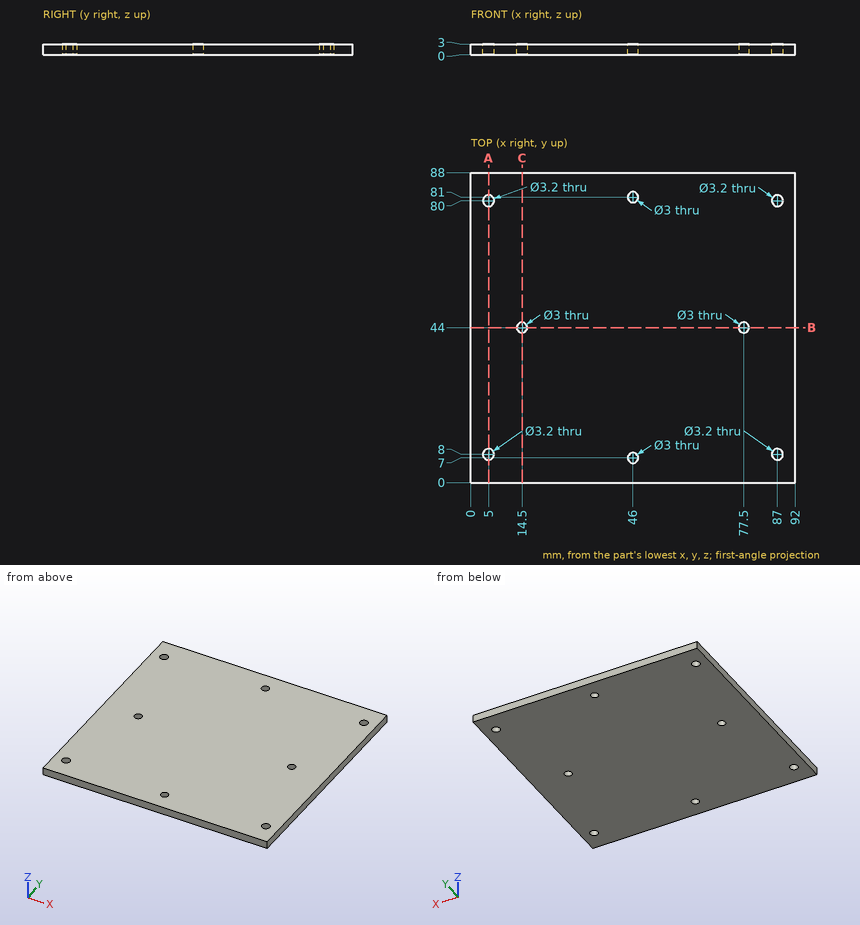
Can you work these out from the drawing? Everything is in mm from the part's minimum corner. Coordinates: 2 decimals unless noted, no trailing zeros. Loops run counter-clockwise (first coordinate to the right, second up) from the corner with the lowest first, then second, coordinate; pieces in that order, holes last. Notation, with made-up numbers: M 36,25 L 56,25 A24 ccw 56,55 Z; hole C 61,69 d3. An arc over 180 degrees is marked long. Put each result on its own line as item: value. Start each with the question number.
(1) Will this pin go through, and if not, where does the flat tip stop? P1, Ø3.5, axis at x = 87, y = 80, coming from the +Z side.
(2) I need wall thicknesses on line 1 (Y direction, x = 46, z = 2.05); line 2 (Y direction, x = 5, z = 2); line 3 (Y direction, x = 77.5, z = 2.45). Which ranges of each line are inside material? Lowest first, please. Write a range as from..to.
(3) Suppose I cut it at B-B on y = 44. Please give me the cut outline in (x, z), then the cut area to 3 significant figures.
(4) Suppose I cut it at A-A on x = 5. Please give me the cut outline in (y, z).
(5) Suppose I cut it at C-C on x = 14.5. Please give me the cut outline in (y, z).
Solutions:
1. P1: stops at z = 3
2. line 1: y = 0..5.5, 8.5..79.5, 82.5..88
2. line 2: y = 0..6.4, 9.6..78.4, 81.6..88
2. line 3: y = 0..42.5, 45.5..88
3. outline: M 0,0 L 13,0 L 13,3 L 0,3 Z; M 16,0 L 76,0 L 76,3 L 16,3 Z; M 79,0 L 92,0 L 92,3 L 79,3 Z
3. area: 258 mm2
4. outline: M 0,0 L 6.4,0 L 6.4,3 L 0,3 Z; M 9.6,0 L 78.4,0 L 78.4,3 L 9.6,3 Z; M 81.6,0 L 88,0 L 88,3 L 81.6,3 Z
5. outline: M 0,0 L 42.5,0 L 42.5,3 L 0,3 Z; M 45.5,0 L 88,0 L 88,3 L 45.5,3 Z
